The listing builds one solid part. Answer for the finished solid, in the listing's coordinates (mm). A direction names the side the tool comes from. Coordinates: 2 decimals unless noted, no trailing zeros. Write each loop counter-clockwise with the first axis right and the second up, starting at its lowest first coordinate (ties: lowest second). Pieces come first, ordered by that corner, then holes.
(1) For a pull along Z with two mould halves and no side action, classify faces 1 (the cylindrical face through (-82.54, 7.57, 70.8)), 2 (the flat face through (-82, 5, 45)), 3 (the flat face through (-1, 5, -1)) as +Z half, -Z half, draft (parallel to the pull), parting line (faces both ways), or undercut.
(2) The part is cut by section C-C on z = -32.5. Determine the outline of the cut face in (x, y).
(3) The part is cut by section B-B on x = -34. Determine the outline of the cut face in (y, z).
(4) Which of the six approach directions +Z, -Z, +X, -X, +Y, -Y give full straight-line access (tool end or side, diameter ignored) to faces 4 (the flat face through (85, 5, 60)), 5 (the flat face through (80, 5, 60)), 6 (the flat face through (-80, 2, -3)), 7 (the flat face through (82, 5, 45))?
(5) Straight lines are drawn through the part: line 1 (Y direction, x = 81.5, z = 72.5); line 2 (Y direction, x = -82, z = 72); line 3 (Z direction, x = 29, y = 2.25). For each, find the intervals that lie inside material, in ascending order.
(6) Given P1, Ø6, axis at x = 7.5, y = 6.5, coming from the -Z side; P2, Ø1.5, axis at x = -83, y = 4, coming from the -Z side; P3, Ø1.5, axis at y = 2.5, z = 18, coming from the +X side; P4, Ø5, axis at x = 8, y = 6.5, coming from the +Z side, each flat-ended and moving along its own axis, determine where each tip first touches the part or whether it passes through.
(7) The part is cut by section A-A on y = 2.5. Determine the outline of the cut face in (x, z).
from build123d import *

# Parameters (mm, degrees)
SKETCH_1_W          = 160
SKETCH_1_H          = 105
EXTRUDE_1_DEPTH     = 5
SKETCH_3_W          = 30.377017425
SKETCH_3_H          = 10
EXTRUDE_3_DEPTH     = 5
SKETCH_4_W          = 30.377017425
SKETCH_4_H          = 10
EXTRUDE_4_DEPTH     = 5
SKETCH_5_R          = 1.7
CUT_EXTRUDE_1_DEPTH = 200
SKETCH_6_R          = 1.7
CUT_EXTRUDE_3_DEPTH = 200
SKETCH_7_R          = 1.7
CUT_EXTRUDE_4_DEPTH = 200


with BuildPart() as part:
    # 草图1 → 凸台-拉伸1 (new body)
    with BuildSketch(Plane(origin=(0, 0, 0), x_dir=(1, 0, 0), z_dir=(0, 1, 0))):
        Rectangle(SKETCH_1_W, SKETCH_1_H)
    extrude(amount=EXTRUDE_1_DEPTH)

    # 草图3 → 凸台-拉伸3 (add)
    with BuildSketch(Plane(origin=(80, 0, 0), x_dir=(0, 0, -1), z_dir=(1, 0, 0))):
        with Locations((-60.188508713, 5)):
            Rectangle(SKETCH_3_W, SKETCH_3_H)
    extrude(amount=EXTRUDE_3_DEPTH)

    # 草图4 → 凸台-拉伸4 (add)
    with BuildSketch(Plane.ZY.offset(80)):
        with Locations((60.188508713, 5)):
            Rectangle(SKETCH_4_W, SKETCH_4_H)
    extrude(amount=EXTRUDE_4_DEPTH)

    # 草图5 → 切除-拉伸1 (cut)
    with BuildSketch(Plane.ZY.offset(80)):
        with Locations((-50, 2.5)):
            Circle(SKETCH_5_R)
    extrude(amount=-CUT_EXTRUDE_1_DEPTH, mode=Mode.SUBTRACT)

    # 草图6 → 切除-拉伸3 (cut)
    with BuildSketch(Plane.ZY.offset(85)):
        with Locations((57.5, 7.5)):
            Circle(SKETCH_6_R)
        with Locations((72.5, 7.5)):
            Circle(SKETCH_6_R)
    extrude(amount=-CUT_EXTRUDE_3_DEPTH, mode=Mode.SUBTRACT)

    # 草图7 → 切除-拉伸4 (cut)
    with BuildSketch(Plane(origin=(85, 0, 0), x_dir=(0, 0, -1), z_dir=(1, 0, 0))):
        with Locations((-72.5, 2.5)):
            Circle(SKETCH_7_R)
    extrude(amount=-CUT_EXTRUDE_4_DEPTH, mode=Mode.SUBTRACT)


solid = part.part
Model answer:
1. face 1: undercut
1. face 2: -Z half
1. face 3: draft
2. outline: (-80, 0) - (80, 0) - (80, 5) - (-80, 5) - close
3. outline: (0, -52.5) - (5, -52.5) - (5, 52.5) - (0, 52.5) - close; hole circle Ø3.4 at (2.5, -50)
4. face 4: +Z, -Z, +X, +Y, -Y
4. face 5: +Z, +Y
4. face 6: -Z, -X, +Y, -Y
4. face 7: -Z, +X, +Y, -Y
5. line 1: y = 0 to 0.8, 4.2 to 5.8, 9.2 to 10
5. line 2: y = 0 to 0.88, 4.12 to 5.88, 9.12 to 10
5. line 3: z = -52.5 to -51.68, -48.32 to 52.5
6. P1: stops at z = -52.5
6. P2: stops at z = 45
6. P3: stops at x = 80
6. P4: stops at z = 52.5
7. outline: (-85, 45) - (-80, 45) - (-80, -48.3) - (80, -48.3) - (80, 45) - (85, 45) - (85, 70.8) - (80, 70.8) - (80, 52.5) - (-80, 52.5) - (-80, 70.8) - (-85, 70.8) - close; (-85, 74.2) - (-80, 74.2) - (-80, 75.38) - (-85, 75.38) - close; (-80, -52.5) - (80, -52.5) - (80, -51.7) - (-80, -51.7) - close; (80, 74.2) - (85, 74.2) - (85, 75.38) - (80, 75.38) - close
